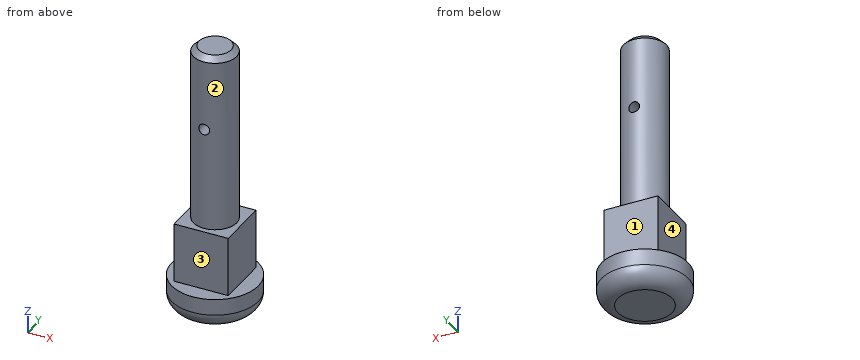
from build123d import *

# Parameters (mm, degrees)
SKETCH1_R                = 8
BOSS_EXTRUDE1_DEPTH      = 6
SKETCH2_W                = 10
SKETCH2_H                = 10
BOSS_EXTRUDE2_DEPTH      = 11
SKETCH4_R                = 4
BOSS_EXTRUDE3_DEPTH      = 44
F_2_0_2_DIAMETER_HOLE1_D = 2
FILLET1_R                = 3
CHAMFER1_SIZE            = 1


with BuildPart() as part:
    # Sketch1 → Boss-Extrude1 (new body)
    with BuildSketch(Plane.XY):
        Circle(SKETCH1_R)
    extrude(amount=-BOSS_EXTRUDE1_DEPTH)

    # Sketch2 → Boss-Extrude2 (add)
    with BuildSketch(Plane.XY):
        Rectangle(SKETCH2_W, SKETCH2_H)
    extrude(amount=BOSS_EXTRUDE2_DEPTH)

    # Sketch4 → Boss-Extrude3 (add)
    with BuildSketch(Plane.XY):
        Circle(SKETCH4_R)
    extrude(amount=BOSS_EXTRUDE3_DEPTH)

    # Ø2.0 (2) Diameter Hole1 (through all)
    with Locations(Plane(origin=(0, 4, 30), x_dir=(1, 0, 0), z_dir=(0, 1, 0))):
        with Locations((0, 0)):
            Hole(F_2_0_2_DIAMETER_HOLE1_D / 2)

    # Fillet1
    fillet1_edges = [part.edges().sort_by_distance(p)[0] for p in [
        (-8, 0, -6),
    ]]
    fillet(fillet1_edges, radius=FILLET1_R)

    # Chamfer1
    chamfer1_edges = [part.edges().sort_by_distance(p)[0] for p in [
        (-4, 0, 44),
    ]]
    chamfer(chamfer1_edges, length=CHAMFER1_SIZE)


solid = part.part
Source: CAD feature listing. Evaluate the final solid. Frame: model axes, mm. Face numbers are marked on the shaded views. A direction names the side the tool comes from. Round coordinates to 2 decimals unless told otherwise and drop trailing zeros. Loops run counter-clockwise (first coordinate to the right, second up) from the corner with the lowest first, then second, coordinate; pieces in that order, holes last.
Q1. First-contact query: P1, Ø8, axis at x = -1.5, y = -5, coming from the +Z side; P2, Ø3, axis at x = -1, z = 3, coming from the -Y side; P3, Ø5, axis at y = -2.5, z = 6, coming from the -X side; P4, Ø5, axis at y = 2.5, z = 34.5, coming from the +X side. Flat tips, straight axial feed; report the tip coordinate or a pass-through.
Q2. Section A-A, the plane y = 0. Return loops of the section in (x, z), plus the area to 3 significant figures.
Q3. Ray query, line 1 (Z direction, x = 0, y = -1.75); line 2 (Y direction, x = 4.75, z = 3); line 3 (X direction, y = -1.5, z = 30). Return the intervals inside material, ascending.
Q4. Access query for the marked faces 1, 2, 3 and 4. Directions: +Z, -Z, +X, -X, +Y, -Y. A direction counts if a zero-diameter tool reaches every point of the face in a straight line with its end or side. Return the directions, or none.
Q5. Section B-B, the plane x = 0. Return loops of the section in (y, z).
Q6. Section D-D, the plane z = 30. Return loops of the section in (x, y), plus the area to 3 significant figures.
Q7. Section C-C, the plane z = 21.5. Return loops of the section in (x, y).
Solutions:
1. P1: stops at z = 44
1. P2: stops at y = -5
1. P3: stops at x = -5
1. P4: stops at x = 4
2. outline: (-8, -3) arc R3 ccw to (-5, -6) - (5, -6) arc R3 ccw to (8, -3) - (8, 0) - (5, 0) - (5, 11) - (4, 11) - (4, 43) - (3, 44) - (-3, 44) - (-4, 43) - (-4, 11) - (-5, 11) - (-5, 0) - (-8, 0) - close; hole circle Ø2 at (0, 30)
2. area: 462 mm2
3. line 1: z = -6 to 29, 31 to 44
3. line 2: y = -5 to 5
3. line 3: x = -3.71 to -1, 1 to 3.71
4. face 1: +Z, +X, -X, +Y
4. face 2: +Z
4. face 3: +Z, +X, -X, -Y
4. face 4: +Z, -X, +Y, -Y
5. outline: (-8, -3) arc R3 ccw to (-5, -6) - (5, -6) arc R3 ccw to (8, -3) - (8, 0) - (5, 0) - (5, 11) - (4, 11) - (4, 29) - (-4, 29) - (-4, 11) - (-5, 11) - (-5, 0) - (-8, 0) - close; (-4, 31) - (4, 31) - (4, 43) - (3, 44) - (-3, 44) - (-4, 43) - close
6. outline: (-1, -3.87) - (-1, 3.87) arc R4 ccw to start; (1, -3.87) arc R4 ccw to (1, 3.87) - close
6. area: 34.4 mm2
7. outline: circle Ø8 at (0, 0)
